```python
from build123d import *

# Parameters (mm, degrees)
F0_W     = 15
F0_H     = 60
F1_DEPTH = 28.5
F3_W     = 56.5
F3_H     = 50
F4_DEPTH = 28.501
F2_W     = 15
F2_H     = 21.875
F5_DEPTH = 12.25
F6_DEPTH = 71.5
F7_DEPTH = 40.751


with BuildPart() as f1:
    # F0 (on Top) → F1 (new body)
    with BuildSketch(Plane.XY):
        Rectangle(F0_W, F0_H)
    extrude(amount=F1_DEPTH)

    # F3 (on face) → F4 (cut, through all)
    with BuildSketch(Plane(origin=(0, 0, 0), x_dir=(1, 0, 0), z_dir=(0, 0, -1))):
        with Locations((35.75, -5)):
            Rectangle(F3_W, F3_H)
    extrude(amount=-F4_DEPTH, mode=Mode.SUBTRACT)

    # F2 (on face) → F5 (join)
    with BuildSketch(Plane.XY.offset(28.5)):
        with Locations((0, 19.0625)):
            Rectangle(F2_W, F2_H)
        with Locations((0, -19.0625)):
            Rectangle(F2_W, F2_H)
    extrude(amount=F5_DEPTH)

    # F5_face (on face) → F6 (join)
    with BuildSketch(Plane(origin=(7.5, 0, 19.11199), x_dir=(0, 1, 0), z_dir=(1, 0, 0))):
        Polygon((-30, -19.11199), (30, -19.11199), (30, 21.63801), (8.125, 21.63801), (8.125, 9.38801), (-8.125, 9.38801), (-8.125, 21.63801), (-30, 21.63801), align=None)
    extrude(amount=F6_DEPTH)

    # F3 (on face) → F7 (cut, through all)
    with BuildSketch(Plane(origin=(0, 0, 0), x_dir=(1, 0, 0), z_dir=(0, 0, -1))):
        with Locations((35.75, -5)):
            Rectangle(F3_W, F3_H)
    extrude(amount=-F7_DEPTH, mode=Mode.SUBTRACT)


solid = f1.part
```
Read the model definition and answer for the solid it produces. Units are mm, in the model's axes. A direction names the side the tool comes from. Give positions to 0.01 mm unless a question says otherwise; leave off trailing zeros. Write each loop counter-clockwise with the first axis right and the second up, starting at its lowest first coordinate (ties: lowest second). Pieces come first, ordered by that corner, then holes. Notation, with made-up numbers: (38.25, 37.5) -> (84.25, 37.5) arc R23 cw to (84.25, 66.5) -> close; hole circle Ø10 at (-22.75, 68.5). An arc over 180 degrees is marked (long way). Answer in a Markdown table with one row per item.
1) Straight lines are drawn through the part: line 1 (X direction, y = -11, z = 36.5); line 2 (Y direction, x = 37, z = 22.5). For each, find the intervals that lie inside material, in ascending order. Write a range as [from, to].
Results list:
| item | result |
|---|---|
| line 1 | [-7.5, 7.5], [64, 79] |
| line 2 | [-30, -20] |
2) A tool of negligible diameter and unlimited length cuts with its end or side. For faces 4 (the flat face through (7.5, 5, 20)), 5 (the flat face through (25.5, -20.4, 0)), 6 (the flat face through (0, 0, 28.5)), from which of +Z, -Z, +X, -X, +Y, -Y can it reach the whole face along a straight path? Write none if from no direction.
Results list:
| item | result |
|---|---|
| face 4 | +Z, -Z, +Y |
| face 5 | -Z, +X, -X, +Y, -Y |
| face 6 | +Z, +X, -X |
3) Section A-A on y = 12.5 is taken. Give the vertices of the cut face in (x, z).
Results list:
| item | result |
|---|---|
| outline | (-7.5, 0) -> (7.5, 0) -> (7.5, 40.75) -> (-7.5, 40.75) -> close; (64, 0) -> (79, 0) -> (79, 40.75) -> (64, 40.75) -> close |
4) Section C-C on x = 3.5 is taken. Give the vertices of the cut face in (y, z) (3 decimals), plus the area to 3 significant figures.
Results list:
| item | result |
|---|---|
| outline | (-30, 0) -> (30, 0) -> (30, 40.75) -> (8.125, 40.75) -> (8.125, 28.5) -> (-8.125, 28.5) -> (-8.125, 40.75) -> (-30, 40.75) -> close |
| area | 2,250 mm^2 |
5) Section B-B on z = 30.5 is taken. Give the vertices of the cut face in (x, y) (3 decimals).
Results list:
| item | result |
|---|---|
| outline | (-7.5, -30) -> (79, -30) -> (79, -8.125) -> (64, -8.125) -> (64, -20) -> (7.5, -20) -> (7.5, -8.125) -> (-7.5, -8.125) -> close; (-7.5, 8.125) -> (7.5, 8.125) -> (7.5, 30) -> (-7.5, 30) -> close; (64, 8.125) -> (79, 8.125) -> (79, 30) -> (64, 30) -> close |
6) Each of these flat-tipped pins is pushed along its axis until it touches: pin 1 Ø12 at (x, y) = (70.5, 1) entering from +Z; pin 2 Ø8 at (x, z) = (43.5, 11) entering from +Y. Where does it stop, or does it pass through?
Results list:
| item | result |
|---|---|
| pin 1 | z = 28.5 |
| pin 2 | y = -20 |
7) Determine the mould class of faces 1 (the flat face through (64, 5, 20)), 2 (the flat face through (35, -30, 21)), 3 (the flat face through (0, 8.125, 35)) for opening direction Y: released by +Y, released by -Y, zero draft, split by the parting line, or undercut.
Results list:
| item | result |
|---|---|
| face 1 | zero draft |
| face 2 | released by -Y |
| face 3 | undercut |
8) Section D-D on z = 8 is taken. Give the vertices of the cut face in (x, y), plus the area to 4 significant figures.
Results list:
| item | result |
|---|---|
| outline | (-7.5, -30) -> (79, -30) -> (79, 30) -> (64, 30) -> (64, -20) -> (7.5, -20) -> (7.5, 30) -> (-7.5, 30) -> close |
| area | 2,365 mm^2 |
